from build123d import *

# Parameters (mm, degrees)
BOSS_EXTRUDE1_DEPTH = 19.05
CHAMFER1_SIZE       = 5.08
SKETCH2_R           = 4
CUT_EXTRUDE1_DEPTH  = 12.7
CIRPATTERN1_COUNT   = 3


with BuildPart() as part:
    # Sketch1 → Boss-Extrude1 (new body)
    with BuildSketch(Plane(origin=(0, 0, 0), x_dir=(1, 0, 0), z_dir=(0, 1, 0))):
        Polygon((40.327916303, -69.85), (80.655832606, 0), (40.327916303, 69.85), (-40.327916303, 69.85), (-80.655832606, 0), (-40.327916303, -69.85), align=None)
    extrude(amount=BOSS_EXTRUDE1_DEPTH)

    # Chamfer1
    chamfer1_edges = [part.edges().sort_by_distance(p)[0] for p in [
        (60.491874454, 19.05, -34.925),
        (0, 19.05, -69.85),
        (-60.491874454, 19.05, -34.925),
        (-60.491874454, 19.05, 34.925),
        (0, 19.05, 69.85),
        (-60.491874454, 0, 34.925),
        (-60.491874454, 0, -34.925),
        (0, 0, -69.85),
        (60.491874454, 0, -34.925),
        (60.491874454, 0, 34.925),
        (0, 0, 69.85),
        (60.491874454, 19.05, 34.925),
    ]]
    chamfer(chamfer1_edges, length=CHAMFER1_SIZE)

    # Sketch2 → Cut-Extrude1 (cut)
    with BuildSketch(Plane(origin=(-60.491874454, 0, 34.925), x_dir=(0.5000000000000001, 0, 0.8660254037844386), z_dir=(-0.8660254037844386, 0, 0.5000000000000001))):
        with Locations((0, 9.525)):
            Circle(SKETCH2_R)
    cut_extrude1 = extrude(amount=-CUT_EXTRUDE1_DEPTH, mode=Mode.SUBTRACT)

    # CirPattern1: Cut-Extrude1 ×3 about axis
    cirpattern1_axis = Axis((0, 0, 0), (0, 1, 0))
    for i in range(1, CIRPATTERN1_COUNT):
        add(cut_extrude1.rotate(cirpattern1_axis, i * 360 / CIRPATTERN1_COUNT), mode=Mode.SUBTRACT)


solid = part.part
Check sheet for the modelled part. Datum: model origin and axes. Units: mm. Round coordinates to 2 decimals unless told otherwise and drop trailing zeros. Loops run counter-clockwise (first coordinate to the right, second up) from the corner with the lowest first, then second, coordinate; pieces in that order, holes last. Notation, with made-up numbers: (7.25, 30.5) - (40.25, 30.5) arc R14 cw to (40.25, 45.5) - close; hole circle Ø5 at (87.5, 34.5). An arc over 180 degrees is marked (long way). Answer as CSV lines item,"result". Start each with the question number.
Item 1: Section check C-C (y = 7.25). Record the boundary of the cut face in (x, z).
Item 2: Scan lines: line 1 (Y direction, x = 0, z = -63.25) (3 decimals); line 2 (Z direction, x = -28, y = 14); line 3 (Y direction, x = 0, z = -67) (3 decimals). Record each from-to range of solid material in increasing order. Write a range as [from, to].
Item 3: Release check for a two-part mould opening along X. For faces 1 (the flat face through (58.54, 2.5, -33.15)), 2 (the flat face through (0.56, 16.55, -67.27)), 3 (the flat face through (-49.52, 9.58, 28.53)), 4 (the flat face through (-58.54, 16.55, 33.15)) record: +X half, -X half, draft (parallel to the pull), parting line (faces both ways), or undercut.
Item 4: Section check D-D (z = 29.5). Count the separate pieces of the cut face and the enclosed holes in it, and give its area (3 significant figures).
Item 5: Depth check by flat-ended pin: P1, Ø4, axis at x = -51, y = 10.5, coming from the -Z side; P2, Ø3, axis at x = 20, y = 15.5, coming from the +Z side; P3, Ø6, axis at y = 17, z = -12, coming from the -X side. Enter the tip coordinate at first touch or a pass-through.
Item 6: Section check A-A (x = 0). Record the boundary of the cut face in (y, z) (3 decimals).
Item 7: Section check B-B (z = 58.5). Record the boundary of the cut face in (x, y).
Report:
1,outline,"(-80.66, 0) - (-40.33, -69.85) - (-3.29, -69.85) - (-3.29, -57.15) - (3.29, -57.15) - (3.29, -69.85) - (40.33, -69.85) - (80.66, 0) - (62.14, 32.08) - (51.14, 25.73) - (47.85, 31.42) - (58.85, 37.77) - (40.33, 69.85) - (-40.33, 69.85) - (-58.85, 37.77) - (-47.85, 31.42) - (-51.14, 25.73) - (-62.14, 32.08) - close"
2,line 1,"y = [0, 5.525], [13.525, 19.05]"
2,line 2,"z = [-69.82, 69.82]"
2,line 3,"y = [2.23, 5.525], [13.525, 16.82]"
3,face 1,"+X half"
3,face 2,"draft"
3,face 3,"undercut"
3,face 4,"-X half"
4,separate pieces,"1"
4,enclosed holes,"2"
4,area,"2,230 mm2"
5,P1,"stops at z = -54.83"
5,P2,"stops at z = 69.82"
5,P3,"stops at x = -74.1"
6,outline,"(0, -64.77) - (5.08, -69.85) - (5.525, -69.85) - (5.525, -57.15) - (13.525, -57.15) - (13.525, -69.85) - (13.97, -69.85) - (19.05, -64.77) - (19.05, 64.77) - (13.97, 69.85) - (5.08, 69.85) - (0, 64.77) - close"
7,outline,"(-46.88, 5.08) - (-41.01, 0) - (41.01, 0) - (46.88, 5.08) - (46.88, 13.97) - (41.01, 19.05) - (-41.01, 19.05) - (-46.88, 13.97) - close"
